Autodesk Inventor part; units mm, degrees
ref_plane "Work Plane1" through (-30.2, 19, -10) normal (1, 0, 0) x (0, 0, -1)
ref_plane "YZ Plane" through (0, 0, 0) normal (1, 0, 0) x (0, 1, 0)
ref_plane "XZ Plane" through (0, 0, 0) normal (0, 1, 0) x (-1, 0, 0)
sketch "Sketch1" plane through (0, 0, 0) normal (0, 1, 0) x (-1, 0, 0)
  line L0 (0, 0) -> (40.2, 0)
  line L1 (40.2, 0) -> (40.2, -155.2)
  line L2 (40.2, -155.2) -> (0, -155.2)
  line L3 (0, -155.2) -> (0, 0)
  line L4 (0, -20) -> (20.2, -20)
  line L5 (20.2, -20) -> (20.2, -135.2)
  line L6 (20.2, -135.2) -> (0, -135.2)
  line L7 (0, -135.2) -> (0, -20)
  line L8 (10.1, -135.2) -> (10.1, -20) construction
  line L9 (20.2, -77.6) -> (0, -77.6) construction
  circle A0 centre (10.1, -77.6) radius 3.5
  line L10 (0, -54.6) -> (20.2, -54.6) construction
  line L11 (20.2, -31.6) -> (0, -31.6) construction
  circle A1 centre (10.1, -54.6) radius 3.5
  circle A2 centre (10.1, -31.6) radius 3.5
  circle A3 centre (10.1, -100.6) radius 3.5
  circle A4 centre (10.1, -123.6) radius 3.5
  line L12 (40.2, -155.2) -> (20.2, -135.2) construction
  line L13 (30.2, -155.2) -> (30.2, 0) construction
  line L14 (20.2, -20) -> (40.2, 0) construction
  circle A5 centre (30.2, -145.2) radius 2.6
  circle A6 centre (30.2, -10) radius 2.6
  circle A7 centre (30.2, -77.6) radius 2.6
  point P0 (0, -135.2)
  dimension "d0" = 115.2
  dimension "d1" = 20.2
  dimension "d2" = 7
  dimension "d3" = 23
  dimension "d4" = 23
  dimension "d11" = 20
  dimension "d12" = 20
  dimension "d13" = 20
  dimension "d14" = 5.2
extrude "Extrusion1" add sketch "Sketch1" along normal blind 12 contours L4 L5 L6 L3
extrude "Extrusion2" add sketch "Sketch1" along normal blind 2 contours A0 | A1 | A2 | A3 | A4
extrude "Extrusion3" add sketch "Sketch1" along normal blind 19 contours L0 L1 L2 L3 L6 L5 L4
sketch "Sketch2" plane through (0, 19, 0) normal (0, 1, 0) x (1, 0, 0)
  line L0 (-40.2, 155.2) -> (-40.2, 0)
  line L1 (-40.2, 0) -> (0, 0)
  line L2 (0, 0) -> (0, 20)
  line L3 (0, 20) -> (-20.2, 20)
  line L4 (-20.2, 20) -> (-20.2, 135.2)
  line L5 (-20.2, 135.2) -> (0, 135.2)
  line L6 (0, 135.2) -> (0, 155.2)
  line L7 (0, 155.2) -> (-40.2, 155.2)
  circle A0 centre (-30.2, 77.6) radius 2.6
  circle A1 centre (-30.2, 145.2) radius 2.6
  circle A2 centre (-30.2, 10) radius 2.6
  line L8 (-30.2, 10) -> (-30.2, 145.2)
ref_plane "Work Plane1" through (-30.2, 19, -10) normal (1, 0, 0) x (0, 0, -1)
mirror "Mirror1" about plane through (-30.2, 19, -10) normal (1, 0, 0) of "Extrusion3", "Extrusion2", "Extrusion1"
equation "\"d1\" = screwTabWidth + tolerance"
equation "\"d2\" = insertDiameter"
equation "\"d11\" = screwTabWidth"
equation "\"d12\" = screwTabWidth"
equation "\"d13\" = screwTabWidth"
equation "\"d14\" = screwDiameter + tolerance"
equation "\"d5\" = insertPadding + insertLength"
equation "\"d7\" = insertPadding"
equation "\"d9\" = insertLength + insertPadding + baseThickness"
equation "\"insertDiameter\" = 7"
equation "\"insertLength\" = 10"
equation "\"insertPadding\" = 2"
equation "\"tolerance\" = 0.2"
equation "\"cellSpacing_1\" = 1"
equation "\"screwDiameter_1\" = 5"
equation "\"baseThickness_1\" = 7"
equation "\"tabThickness_1\" = 0.8"
equation "\"batteryBoxWidth\" = 162"
equation "\"sheetMetalThickness\" = 3.175"
properties part number "CO-1-1-CellSpacerMountMiddle"
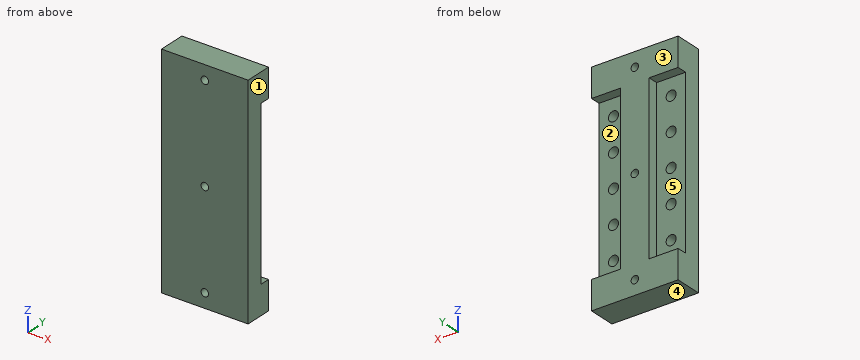
For this review, take the finished solid that the model builds, in its own axes (mm). Face numbers are marked on the shaded views. A direction names the side the tool comes from. Coordinates: 2 decimals unless noted, no trailing zeros. Write each loop counter-clockwise with the first axis right and the second up, starting at its lowest first coordinate (ties: lowest second). Pieces come first, ordered by that corner, then holes. Notation, with made-up numbers: (-10, -11.75) - (8, -11.75) arc R8 cw to (8, 3.25) - close; hole circle Ø4 at (11.25, 33.5). An arc over 180 degrees is marked (long way). Put each result on its own line as item: value.
1. Add section C-C, the plane z = -100.6. Give the boundary of the cut face in (x, y).
Values found:
outline: (-60.4, 0) - (0, 0) - (0, 12) - (-6.6, 12) - (-6.6, 2) - (-13.6, 2) - (-13.6, 12) - (-20.2, 12) - (-20.2, 19) - (-40.2, 19) - (-40.2, 12) - (-46.8, 12) - (-46.8, 2) - (-53.8, 2) - (-53.8, 12) - (-60.4, 12) - close
2. Add section B-B, the plane z = -10. Give the boundary of the cut face in (x, y), then the cut area to 3 significant figures.
Values found:
outline: (-60.4, 0) - (-32.8, 0) - (-32.8, 19) - (-60.4, 19) - close; (-27.6, 0) - (0, 0) - (0, 19) - (-27.6, 19) - close
area: 1,050 mm²
3. Add section A-A, the plane y = 6.5. Count the separate pieces of the cut face and the enclosed holes in it, then the cut area to 3 significant figures.
Values found:
separate pieces: 1
enclosed holes: 13
area: 8,930 mm²
4. Machinability: for the marked faces 1 and 2, which of the approach directions +Z, -Z, +X, -X, +Y, -Y give a long, thin tool a straight path to every point of the face, cutting with its end or side? Answer none if there is none.
Values found:
face 1: +Z, -Z, +X, +Y, -Y
face 2: +X, +Y
5. Add section D-D, the plane x = -45. Give the boundary of the cut face in (y, z).
Values found:
outline: (0, -155.2) - (19, -155.2) - (19, -135.2) - (12, -135.2) - (12, -20) - (19, -20) - (19, 0) - (0, 0) - close
6. For pin 1 (2 mm diameter, centred on x = -50.5, z = -55, fed in from +Y); pin 2 (9 mm diameter, centred on x = -10.1, z = -54.6, fed in from +Y); pin 3 (3.5 mm diameter, centred on y = 14, z = -97.5, fed in from -X), all flat-tipped, find the tip position at first contact; note any pin that passes through.
Values found:
pin 1: y = 2
pin 2: y = 12
pin 3: x = -40.2
7. Mouldability with a two-part tool opening along Z and no side actions: class the marked faces 3, 4 and 5 as released by +Z, released by -Z, zero draft, split by the parting line, or undercut.
Values found:
face 3: zero draft
face 4: released by -Z
face 5: undercut
8. Wall thickness on probe 1 along Z at (x, y) = (-50.3, 5.25); probe 2 along X at (y, z) = (13, -10); probe 3 along Z at (x, y) = (-8, 15.5): over which ranges is each line inside the solid? List them lowest first.
Values found:
probe 1: -155.2 to -127.1, -120.1 to -104.1, -97.1 to -81.1, -74.1 to -58.1, -51.1 to -35.1, -28.1 to 0
probe 2: -60.4 to -32.8, -27.6 to 0
probe 3: -155.2 to -135.2, -20 to 0
